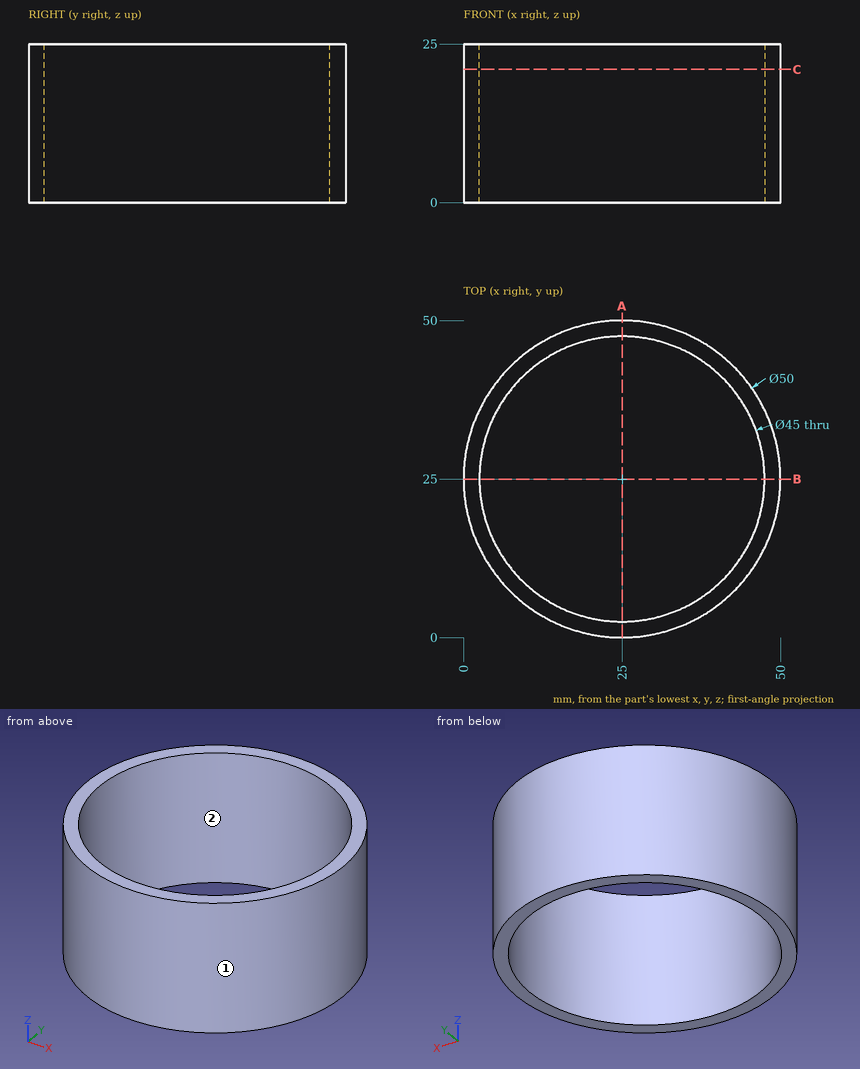
Source: three-view drawing plus pictorial views. Frame: mm from the lowest corner of the part. Give positions to 0.01 mm unless a question says otherwise; leave off trailing zeros. Loops run counter-clockwise (first coordinate to the right, second up) from the corner with the lowest first, then second, coordinate; pieces in that order, holes last. Notation, with made-up numbers: M 16.25,17 L 56.25,17 A15 cw 56.25,42 Z; hole C 43.25,57 d6. An arc over 180 degrees is marked long. Put each result on its own line as item: value.
Q1. Mould query, pull axis Y, two halves, no side actions, for the marked faces 1 and 2. Classes: released by +Y, released by -Y, zero draft, split by the parting line, or undercut.
Response values:
face 1: split by the parting line
face 2: undercut
Q2. Section C-C (z = 21). Return the cut outline in (x, y).
Response values:
outline: C 25,25 d50; hole C 25,25 d45
Q3. Line query: probe 1 along Y at (x, z) = (25, 10); probe 2 along X at (y, z) = (24.5, 15.5) (3 decimals); probe 3 along Y at (x, z) = (7, 13.75). Output: solid intervals per line, ascending. Write a range as [from, to].
Response values:
probe 1: y = [0, 2.5], [47.5, 50]
probe 2: x = [0.005, 2.506], [47.494, 49.995]
probe 3: y = [7.65, 11.5], [38.5, 42.35]
Q4. Pin query (flat end, axial travel): P1, Ø1.5, axis at y = 11.5, z = 11, coming from the +X side; P2, Ø1, axis at y = 30, z = 17, coming from the -X side; P3, Ø1, axis at x = 33.5, y = 44, coming from the -Z side; P4, Ø1.5, axis at y = 32, z = 3, coming from the -X side. Return the tip coordinate at first contact, or that it passes through.
Response values:
P1: stops at x = 46.5
P2: stops at x = 0.41
P3: passes through
P4: stops at x = 0.79
Q5. Section A-A (x = 25). Return the cut outline in (y, z), and give its area (3 significant figures).
Response values:
outline: M 0,0 L 2.5,0 L 2.5,25 L 0,25 Z; M 47.5,0 L 50,0 L 50,25 L 47.5,25 Z
area: 125 mm²
